For this review, take the finished solid that the model builds, in its own axes (mm). A direction names the side the tool comes from. Coordinates: 2 decimals unless noted, no trailing zeros. Write each loop counter-clockwise with the first axis right and the second up, starting at its lowest first coordinate (ties: lowest second). Pieces come first, ordered by that corner, then holes. Notation, with made-up numbers: (39.5, 10) - (68.5, 10) arc R30 ccw to (68.5, 42) - close; hole circle Ø5 at (59, -6). An arc over 180 degrees is marked (long way). Write each question's results on one line, items separated by ' | '.
from build123d import *

# Parameters (mm, degrees)
EXTRUDE_1_DEPTH          = 7.5
CUT_EXTRUDE_1_DEPTH      = 45.584481316
CUT_EXTRUDE_1_DEPTH_BACK = 45.584481316
SKETCH_2_R               = 4.2
CUT_EXTRUDE_2_DEPTH      = 51.621141828
CUT_EXTRUDE_2_DEPTH_BACK = 51.621141828
SKETCH_3_R               = 4.2
FILLET_1_R               = 3
SKETCH_4_R               = 4.2
SKETCH_4_R_2             = 3.5
EXTRUDE_2_DEPTH          = 0.8
SKETCH_5_R               = 4.2
SKETCH_5_R_2             = 3.5
EXTRUDE_3_DEPTH          = 0.8


with BuildPart() as part:
    # ｽｹｯﾁ1 → ﾎﾞｽ - 押し出し1 (new, symmetric)
    with BuildSketch(Plane.XY):
        Polygon((0, 0), (-24.445436483, 24.445436483), (-20.909902577, 27.980970389), (2.071067812, 5), (16.213203436, 5), (30.355339059, 19.142135624), (33.890872965, 15.606601718), (18.284271247, 0), align=None)
    extrude(amount=EXTRUDE_1_DEPTH, both=True)

    # ｽｹｯﾁ2 → ｶｯﾄ - 押し出し1 (cut, two sides: drawn at the far end of the back side and taken through both)
    with BuildSketch(Plane(origin=(0, 0, 0), x_dir=(0, 0, 1), z_dir=(-0.7071067811865487, -0.7071067811865464, 0)).offset(-CUT_EXTRUDE_1_DEPTH_BACK)):
        with Locations(Location((0, 27.071067812, 0), (0, 0, 270))):
            Circle(SKETCH_2_R)
    extrude(amount=CUT_EXTRUDE_1_DEPTH + CUT_EXTRUDE_1_DEPTH_BACK, mode=Mode.SUBTRACT)

    # ｽｹｯﾁ3 → ｶｯﾄ - 押し出し2 (cut, two sides: drawn at the far end of the back side and taken through both)
    with BuildSketch(Plane(origin=(9.142135624, -9.142135624, 0), x_dir=(0, 0, -1), z_dir=(0.707106781186549, -0.7071067811865461, 0)).offset(-CUT_EXTRUDE_2_DEPTH_BACK)):
        with Locations(Location((0, 27.5, 0), (0, 0, 90))):
            Circle(SKETCH_3_R)
    extrude(amount=CUT_EXTRUDE_2_DEPTH + CUT_EXTRUDE_2_DEPTH_BACK, mode=Mode.SUBTRACT)

    # ﾌｨﾚｯﾄ1
    fillet_1_edges = [part.edges().sort_by_distance(p)[0] for p in [
        (32.123106012, 17.374368671, -7.5),
        (32.123106012, 17.374368671, 7.5),
        (0, 0, 0),
        (2.071067812, 5, 0),
        (16.213203436, 5, 0),
        (18.284271247, 0, 0),
        (-22.67766953, 26.213203436, 7.5),
        (-22.67766953, 26.213203436, -7.5),
    ]]
    fillet(fillet_1_edges, radius=FILLET_1_R)

    # ｽｹｯﾁ4 → ﾎﾞｽ - 押し出し2 (add)
    with BuildSketch(Plane(origin=(0, 0, 0), x_dir=(0, 0, -1), z_dir=(0.7071067811865475, 0.7071067811865476, 0))):
        with Locations(Location((0, 27.071067812, 0), (0, 0, 270))):
            Circle(SKETCH_4_R)
        with Locations(Location((0, 27.071067812, 0), (0, 0, 90))):
            Circle(SKETCH_4_R_2, mode=Mode.SUBTRACT)
    extrude(amount=EXTRUDE_2_DEPTH)

    # ｽｹｯﾁ5 → ﾎﾞｽ - 押し出し3 (add)
    with BuildSketch(Plane(origin=(9.142135624, -9.142135624, 0), x_dir=(0, 0, 1), z_dir=(-0.7071067811865485, 0.7071067811865467, 0))):
        with Locations(Location((0, 27.5, 0), (0, 0, 90))):
            Circle(SKETCH_5_R)
        with Locations(Location((0, 27.5, 0), (0, 0, 270))):
            Circle(SKETCH_5_R_2, mode=Mode.SUBTRACT)
    extrude(amount=EXTRUDE_3_DEPTH)


solid = part.part
Q1. Take a section at A-A on z = 1.5. State the section outline as (x, y) points (1 decimal).
Results found:
outline: (-24.4, 24.4) - (-21.4, 21.4) - (-20.8, 21.9) - (-21.4, 22.5) - (-18.4, 25.5) - (-20.9, 28) - close; (-16.9, 16.9) - (-0.9, 0.9) arc R3 ccw to (1.2, 0) - (17, 0) arc R3 ccw to (19.2, 0.9) - (26.4, 8.1) - (25.8, 8.6) - (25.2, 8.1) - (22.3, 11.1) - (17.1, 5.9) arc R3 cw to (15, 5) - (3.3, 5) arc R3 cw to (1.2, 5.9) - (-12.8, 19.9) - (-15.8, 16.9) - (-16.3, 17.5) - close; (27.8, 16.6) - (30.8, 13.6) - (30.3, 13.1) - (30.8, 12.5) - (33.9, 15.6) - (30.4, 19.1) - close
Q2. Take a section at B-B on y = 7. State the section outline as (x, z) points.
Results found:
outline: (-7, -7.5) - (0.07, -7.5) - (0.07, 7.5) - (-7, 7.5) - close; (18.21, -7.5) - (25.28, -7.5) - (25.28, 7.5) - (18.21, 7.5) - close
Q3. Take a section at C-C on z = 5.25. State the section outline as (x, y) points, plus the area to 3 significant figures.
Results found:
outline: (-24.38, 24.38) - (-0.88, 0.88) arc R3 ccw to (1.24, 0) - (17.04, 0) arc R3 ccw to (19.16, 0.88) - (33.82, 15.54) - (30.29, 19.07) - (17.09, 5.88) arc R3 cw to (14.97, 5) - (3.31, 5) arc R3 cw to (1.19, 5.88) - (-20.84, 27.91) - close | area: 353 mm2
Q4. Mouldability with a two-part tool opening along Z and no side actions: class faces 3 (the face through (32.1, 17.4, 0.1)), 4 (the face through (3, 4, -7.5)), 5 (the face through (3, 4, 7.5)), 6 (the face through (-14.24, 18.38, 1.26)) as pulls with the +Z half, pulls with the -Z half, needs draft (parallel to the pull), parting line crosses it, or undercut.
Results found:
face 3: needs draft | face 4: pulls with the -Z half | face 5: pulls with the +Z half | face 6: undercut
Q5. Wall thickness on line 1 along Y through (x, z) = (11, 0.25); line 2 along X through (y, z) = (5.75, 5.75); line 3 along X through (y, z) = (18, 0.5): over which ranges is each line inside the solid? List them lowest first. Write a range as from..to.
Results found:
line 1: 0..5 | line 2: -5.75..1.33, 16.95..24.03 | line 3: -14.39..-10.93, 29.21..31.5
Q6. Take a section at D-D on x = 11. State the section outline as (y, z) points.
Results found:
outline: (0, -7.5) - (5, -7.5) - (5, 7.5) - (0, 7.5) - close
Q7. For faces 1 (the face through (0.079, 0.235, 0.105)), 2 (the face through (22.157, 10.944, 1.772)), list the 3-axis set-ups (+Z, -Z, +X, -X, +Y, -Y) from which the entire face can be reached by the end or side of a thin tool; tool diameter is ignored.
Results found:
face 1: +Z, -Z, -X, -Y | face 2: +Z, -Z, +Y
Q8. For pin 1 (1.5 mm diameter, centred on x = 0.5, z = -3, fed in from +Y); pin 2 (4 mm diameter, centred on y = 10, z = 4, fed in from -X); pin 3 (3 mm diameter, centred on x = 9, z = 5, fed in from +Y), all flat-tipped, find the tip position at first contact; note any pin that passes through.
Results found:
pin 1: y = 7.32 | pin 2: x = -12 | pin 3: y = 5
